```python
from build123d import *

# Parameters (mm, degrees)
F0_W     = 100.2
F0_H     = 45.2
F1_DEPTH = 30
F3_DEPTH = 105.001
F6_DEPTH = 105
F4_W     = 72.2
F4_H     = 25.1
F4_R     = 1.5
F7_DEPTH = 5
F8_DEPTH = 5


with BuildPart() as f1:
    # F0 (on Top) → F1 (new body)
    with BuildSketch(Plane.XY):
        Polygon((52.5, 25), (-52.5, 25), (-52.5, 4), (-52.5, -4), (-52.5, -25), (52.5, -25), (52.5, -4), (52.5, 4), align=None)
        Rectangle(F0_W, F0_H, mode=Mode.SUBTRACT)
    extrude(amount=F1_DEPTH)

    # F2 (on face) → F3 (cut, through all)
    with BuildSketch(Plane.YZ.offset(52.5)):
        Polygon((-25, 12), (25, 30), (-25, 30), align=None)
    extrude(amount=-F3_DEPTH, mode=Mode.SUBTRACT)

    # F5 (on face) → F6 (join)
    with BuildSketch(Plane(origin=(-52.5, 0, 0), x_dir=(0, -1, 0), z_dir=(-1, 0, 0))):
        Polygon((25, 12), (-25, 30), (-25, 28.0869124432), (25, 10.0869124432), align=None)
    extrude(amount=-F6_DEPTH)

    # F4 (on face) → F7 (cut)
    with BuildSketch(Plane(origin=(0, -6.6926345609, 18.5906515581), x_dir=(1, 0, 0), z_dir=(0, -0.3387194683, 0.9408874119))):
        with Locations((1.5, 5.7432311296)):
            Rectangle(F4_W, F4_H)
        with Locations((39.1, -9.9067688704)):
            Circle(F4_R)
        with Locations((39.1, 21.2932311296)):
            Circle(F4_R)
        with Locations((-36.1, -9.9067688704)):
            Circle(F4_R)
        with Locations((-36.1, 21.2932311296)):
            Circle(F4_R)
    extrude(amount=-F7_DEPTH, mode=Mode.SUBTRACT)

    # F5 (on face) → F8 (cut)
    with BuildSketch(Plane(origin=(-52.5, 0, 0), x_dir=(0, -1, 0), z_dir=(-1, 0, 0))):
        Polygon((-3.4536782682, 11.6150599721), (-17.5669894462, 16.6958519962), (-18.9218673193, 12.9323023487), (-4.8085561413, 7.8515103246), align=None)
    extrude(amount=-F8_DEPTH, mode=Mode.SUBTRACT)


solid = f1.part
```
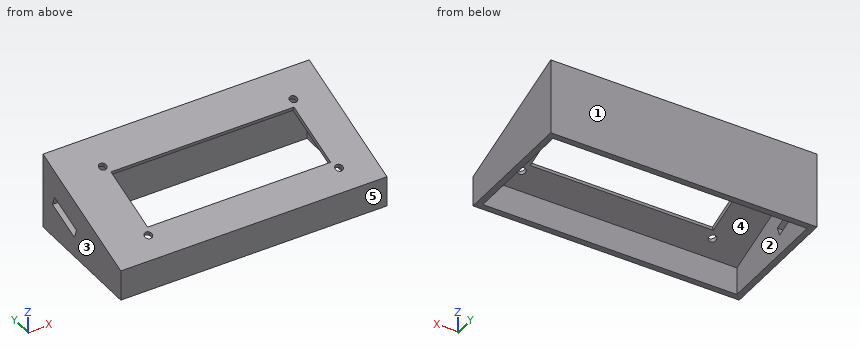
The listing builds one solid part. Answer for the finished solid, in the listing's coordinates (mm). Face numbers are marked on the shaded views. A direction names the side the tool comes from. Give positions to 0.01 mm unless a question says otherwise; leave off trailing zeros. Write each loop counter-clockwise with the first axis right and the second up, starting at its lowest first coordinate (ties: lowest second). Pieces come first, ordered by that corner, then holes. Notation, with made-up numbers: (28.25, 52) -> (52.25, 52) arc R5 cw to (52.25, 59) -> close; hole circle Ø5 at (62.25, -9.5). An arc over 180 degrees is marked (long way). Use one line per item in the form item = value.
1) Section A-A on x = 30 is taken. Write down the section's boundary in (y, z), plus the area to 3 significant figures.
Result:
outline = (-25, 0) -> (-22.6, 0) -> (-22.6, 10.95) -> (-12.49, 14.59) -> (-13.1, 16.29) -> (-25, 12) -> close; (10.52, 24.79) -> (11.13, 23.09) -> (22.6, 27.22) -> (22.6, 0) -> (25, 0) -> (25, 30) -> close
area = 142 mm²
2) Section B-B on y = 9.5 is taken. Write down the section's boundary in (x, z).
Result:
outline = (-52.5, 0) -> (-50.1, 0) -> (-50.1, 9.54) -> (-52.5, 9.54) -> close; (-52.5, 13.79) -> (-50.1, 13.79) -> (-50.1, 22.51) -> (-34.6, 22.51) -> (-34.6, 24.42) -> (-52.5, 24.42) -> close; (37.6, 22.51) -> (50.1, 22.51) -> (50.1, 0) -> (52.5, 0) -> (52.5, 24.42) -> (37.6, 24.42) -> close
3) Each of these flat-tipped pins is pushed along its axis until it touches: P1, Ø1.5, axis at x = -29, y = 14, coming from the +Z side; P2, Ø10, axis at x = 31.5, y = 14, coming from the +Z side. Where does it stop, or does it pass through?
Result:
P1 = 26.31
P2 = 27.84
4) Straight lines are drawn through the part: probe 1 along X at (y, z) = (-3, 4.5); probe 2 along Y at (x, z) = (-29, 1.5); probe 3 along Y at (x, z) = (-11.5, 22.5). For each, find the intervals that lie inside material, in ascending order.
Result:
probe_1 = -52.5 to -50.1, 50.1 to 52.5
probe_2 = -25 to -22.6, 22.6 to 25
probe_3 = 22.6 to 25
5) Section D-D on y = 1.5 is taken. Write down the section's boundary in (x, z), plus the area to 3 significant figures.
Result:
outline = (-52.5, 0) -> (-50.1, 0) -> (-50.1, 19.63) -> (-34.6, 19.63) -> (-34.6, 21.54) -> (-52.5, 21.54) -> close; (37.6, 19.63) -> (50.1, 19.63) -> (50.1, 0) -> (52.5, 0) -> (52.5, 21.54) -> (37.6, 21.54) -> close
area = 157 mm²
6) Section C-C on z = 6.25 is taken. Write down the section's boundary in (x, y).
Result:
outline = (-52.5, -25) -> (52.5, -25) -> (52.5, 25) -> (-52.5, 25) -> close; hole (-50.1, -22.6) -> (50.1, -22.6) -> (50.1, 22.6) -> (-50.1, 22.6) -> close
7) A tool of negligible diameter and unlimited length cuts with its end or side. For the marked faces 4 and 5, from which of +Z, -Z, +X, -X, +Y, -Y can it reach the whole face along a straight path? Write none if from no direction.
Result:
face_4 = -Z
face_5 = +Z, -Z, +X, -X, -Y
8) For a pull along X with two mould halves and no side action, classify the marked faces 1, 2 and 3 as +X half, -X half, draft (parallel to the pull), parting line (faces both ways), or undercut.
Result:
face_1 = draft
face_2 = undercut
face_3 = -X half
